```python
from build123d import *

# Parameters (mm, degrees)
SKETCH_6_R      = 40
EXTRUDE_1_DEPTH = 3
EXTRUDE_2_DEPTH = 1


with BuildPart() as part:
    # 草图6 → 凸台-拉伸1 (new body)
    with BuildSketch(Plane(origin=(0, 0, 0), x_dir=(1, 0, 0), z_dir=(0, 1, 0))):
        with Locations(Location((19.514251299, 24.77976127, 0), (0, 0, 270))):
            Circle(SKETCH_6_R)
    extrude(amount=-EXTRUDE_1_DEPTH)

    # 草图5 → 凸台-拉伸2 (add)
    with BuildSketch(Plane(origin=(0, 0, 0), x_dir=(1, 0, 0), z_dir=(0, 1, 0))):
        with BuildLine():
            Line((-0.848561441, 11.65053417), (10.884604209, 11.65053417))
            Line((10.884604209, 11.65053417), (14.304935387, 24.086135056))
            Line((14.304935387, 24.086135056), (29.829988347, 24.086135056))
            add(Edge.make_bspline(
                [(29.829988347, 24.086135056), (31.936484303, 24.4825638), (34.318672471, 25.163188991), (36.899310154, 26.291897866), (41.512516948, 30.702347463), (41.488102133, 36.127500115), (39.148657484, 41.930059677), (35.435285923, 42.747710664), (34.028305284, 45.040203592), (29.903175199, 45.422244415)],
                knots=[0, 0, 0, 0, 0, 0, 0, 0, 0, 0, 1, 1, 1, 1, 1, 1, 1, 1, 1, 1], degree=9))
            Line((29.903175199, 45.422244415), (1.440650879, 45.422244415))
            Line((1.440650879, 45.422244415), (6.750403312, 37.405182946))
            Line((6.750403312, 37.405182946), (11.26337671, 32.626274642))
            Line((11.26337671, 32.626274642), (22.289106818, 32.626274642))
            Line((22.289106818, 32.626274642), (17.706952403, 37.77757749))
            Line((17.706952403, 37.77757749), (28.656556673, 37.77757749))
            add(Edge.make_bspline(
                [(28.656556673, 37.77757749), (30.140944485, 37.467864792), (32.017287649, 36.447603196), (32.240103399, 33.011549778), (30.02639504, 32.225274016), (28.810885255, 31.820229302)],
                knots=[0, 0, 0, 0, 0, 0, 1, 1, 1, 1, 1, 1], degree=5))
            Line((28.810885255, 31.820229302), (6.42710467, 31.820229302))
            Line((6.42710467, 31.820229302), (1.262783116, 12.592072153))
            Line((1.262783116, 12.592072153), (-0.848561441, 11.65053417))
        make_face()
        Polygon((39.877064038, 13.479058766), (30.809384671, 23.309535699), (19.814492322, 23.309535699), (26.172284787, 16.30574677), (17.246103581, 16.30574677), (38.422169227, 5.825267085), (39.049534436, 5.514770865), (31.775865335, 13.552375437), align=None)
    extrude(amount=EXTRUDE_2_DEPTH)


solid = part.part
```
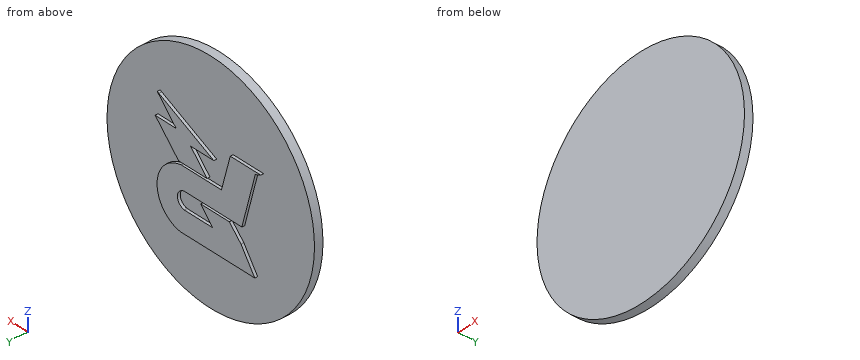
For this review, take the finished solid that the model builds, in its own axes (mm). Coordinates: 2 decimals unless noted, no trailing zeros. Order: outer loops, then holes, each group sorted by start corner. A loop starts at its lowest first (then second) coordinate and runs counter-clockwise, first axis right, second up. Notation, with made-up numbers: (-30.5, 33.5) - (-9.5, 33.5) arc R23 cw to (-9.5, 66.5) - close; hole circle Ø10 at (85, 56). An arc over 180 degrees is marked (long way). Answer as a JSON object with one key per item and string values. Group by question number.
1. We need section B-B on z = -9. State the section outline as (x, y) points, then the cut area to 3 significant figures.
2. We need section A-A on x = 8. State the section outline as (y, z) points.
3. We need section D-D on z = 3.5. State the section outline as (x, y) points, then the cut area to 3 significant figures.
4. Clearance check with flat-ended pins moving along their axes: P1, Ø2, axis at x = 38, y = -0.5, coming from the -Z side; P2, Ø0.8, axis at x = 23, y = 0.5, coming from the +Z side; P3, Ø2, axis at x = -12, z = -48, coming from the +Y side; P4, Ø24, axis at x = 25, z = -7.5, coming from the +Y side. State where each tip first meets the part, or that it passes through.
5. For probe 1 along Y at (x, z) = (48, -10.5); probe 2 along Z at (x, y) = (13, -1.7); probe 3 along X at (y, z) = (-0.9, -45), list the stretches that pass through material, from the lowest coordinate up.
6. We need section C-C on y = -2.35. State the section outline as (x, z) points.
Final values:
{
 "1": {"outline": "(-17.24, -3) - (56.27, -3) - (56.27, 0) - (35.9, 0) - (35.9, 1) - (32.01, 1) - (32.01, 0) - (-17.24, 0) - close", "area": "224 mm²"},
 "2": {"outline": "(-3, -63.09) - (0, -63.09) - (0, -45.42) - (1, -45.42) - (1, -36.08) - (0, -36.08) - (0, -31.82) - (1, -31.82) - (1, -11.65) - (0, -11.65) - (0, 13.53) - (-3, 13.53) - close"},
 "3": {"outline": "(-8.77, -3) - (47.8, -3) - (47.8, 0) - (-8.77, 0) - close", "area": "170 mm²"},
 "4": {"P1": "z = -60.76", "P2": "z = -13.26", "P3": "y = 0", "P4": "y = 1"},
 "5": {"probe 1": "-3 to 0", "probe 2": "-64.25 to 14.69", "probe 3": "-15 to 54.03"},
 "6": {"outline": "circle Ø80 at (19.51, -24.78)"}
}
